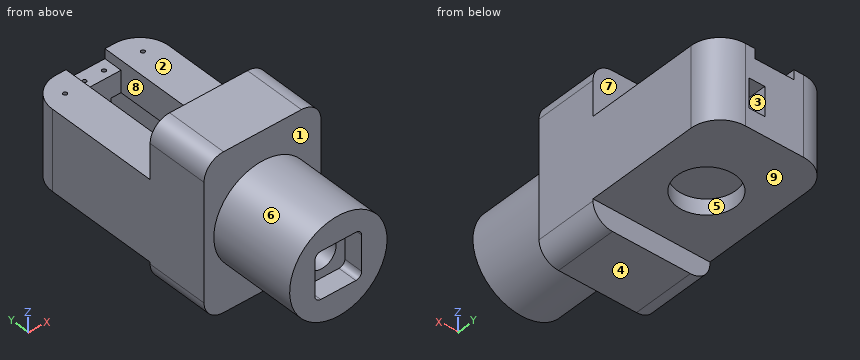
from build123d import *

# Parameters (mm, degrees)
SKETCH1_R                = 25
BOSS_EXTRUDE1_DEPTH      = 45
SKETCH2_W                = 60
SKETCH2_H                = 80
BOSS_EXTRUDE2_DEPTH      = 45
FILLET1_R                = 10
SKETCH3_W                = 60
SKETCH3_H                = 41
BOSS_EXTRUDE3_DEPTH      = 60
SKETCH4_W                = 20
SKETCH4_H                = 41
CUT_EXTRUDE1_DEPTH       = 32
SKETCH5_W                = 20
SKETCH5_H                = 9.5
CUT_EXTRUDE2_DEPTH       = 5
SKETCH7_R                = 15
CUT_EXTRUDE3_DEPTH       = 8
CUT_EXTRUDE4_REACH       = 163.567
SKETCH8_R                = 21
FILLET2_R                = 15
CUT_EXTRUDE5_REACH       = 169.812
SKETCH9_W                = 65
SKETCH9_H                = 65
CUT_EXTRUDE6_REACH       = 163.567
SKETCH10_W               = 65
SKETCH10_H               = 65
SKETCH11_R               = 1
CUT_EXTRUDE7_DEPTH       = 10
SKETCH12_R               = 1
CUT_EXTRUDE8_DEPTH       = 10
CUT_EXTRUDE9_START       = -27
SKETCH13_W               = 10
SKETCH13_H               = 9.5
CUT_EXTRUDE9_DEPTH       = 27
CUT_EXTRUDE10_DEPTH      = 5
CUT_EXTRUDE10_DEPTH_BACK = 3
SKETCH14_W               = 15
SKETCH14_H               = 62.680052408
SKETCH15_R               = 7.5
CUT_EXTRUDE11_DEPTH      = 90
SKETCH16_W               = 24
SKETCH16_H               = 24
CUT_EXTRUDE12_DEPTH      = 10
FILLET3_R                = 3


with BuildPart() as part:
    # Sketch1 → Boss-Extrude1 (new body)
    with BuildSketch(Plane(origin=(0, 0, 0), x_dir=(1, 0, 0), z_dir=(0, 1, 0))):
        with Locations(Location((0, 0, 0), (0, 0, 90))):
            Circle(SKETCH1_R)
    extrude(amount=BOSS_EXTRUDE1_DEPTH)

    # Sketch2 → Boss-Extrude2 (add)
    with BuildSketch(Plane(origin=(0, 45, 0), x_dir=(1, 0, 0), z_dir=(0, 1, 0))):
        Rectangle(SKETCH2_W, SKETCH2_H)
    extrude(amount=BOSS_EXTRUDE2_DEPTH)

    # Fillet1
    fillet1_edges = [part.edges().sort_by_distance(p)[0] for p in [
        (-30, 67.5, -40),
        (-30, 67.5, 40),
        (30, 67.5, 40),
        (30, 67.5, -40),
    ]]
    fillet(fillet1_edges, radius=FILLET1_R)

    # Sketch3 → Boss-Extrude3 (add)
    with BuildSketch(Plane(origin=(0, 90, 0), x_dir=(1, 0, 0), z_dir=(0, 1, 0))):
        with Locations((0, 8.5)):
            Rectangle(SKETCH3_W, SKETCH3_H)
    extrude(amount=BOSS_EXTRUDE3_DEPTH)

    # Sketch4 → Cut-Extrude1 (cut)
    with BuildSketch(Plane.XY.offset(12)):
        with Locations((0, 120)):
            Rectangle(SKETCH4_W, SKETCH4_H)
    extrude(amount=-CUT_EXTRUDE1_DEPTH, mode=Mode.SUBTRACT)

    # Sketch5 → Cut-Extrude2 (cut)
    with BuildSketch(Plane.XY.offset(12)):
        with Locations((0, 94.75)):
            Rectangle(SKETCH5_W, SKETCH5_H)
        with Locations((0, 145.25)):
            Rectangle(SKETCH5_W, SKETCH5_H)
    extrude(amount=-CUT_EXTRUDE2_DEPTH, mode=Mode.SUBTRACT)

    # Sketch7 → Cut-Extrude3 (cut)
    with BuildSketch(Plane(origin=(0, 0, -29), x_dir=(-1, 0, 0), z_dir=(0, 0, -1))):
        with Locations((0.1, 109.5)):
            Circle(SKETCH7_R)
    extrude(amount=-CUT_EXTRUDE3_DEPTH, mode=Mode.SUBTRACT)

    # Sketch8 → Cut-Extrude4 (cut, up to next)
    with BuildSketch(Plane.XY.offset(12), mode=Mode.PRIVATE) as cut_extrude4_sk1:
        with Locations((-0.1, 109.5)):
            Circle(SKETCH8_R)
    cut_extrude4_tool1 = extrude(cut_extrude4_sk1.sketch, amount=CUT_EXTRUDE4_REACH, mode=Mode.PRIVATE) & part.part
    add(cut_extrude4_tool1.solids().sort_by_distance((-0.1, 109.5, 12))[0], mode=Mode.SUBTRACT)

    # Fillet2
    fillet2_edges = [part.edges().sort_by_distance(p)[0] for p in [
        (-30, 150, -8.5),
        (30, 150, -8.5),
    ]]
    fillet(fillet2_edges, radius=FILLET2_R)

    # Sketch9 → Cut-Extrude5 (cut, up to next)
    with BuildSketch(Plane(origin=(0, 0, -29), x_dir=(-1, 0, 0), z_dir=(0, 0, -1)), mode=Mode.PRIVATE) as cut_extrude5_sk1:
        with Locations((0.1, 109.5)):
            Rectangle(SKETCH9_W, SKETCH9_H)
    cut_extrude5_tool1 = extrude(cut_extrude5_sk1.sketch, amount=CUT_EXTRUDE5_REACH, mode=Mode.PRIVATE) & part.part
    add(cut_extrude5_tool1.solids().sort_by_distance((-0.1, 109.5, -29))[0], mode=Mode.SUBTRACT)

    # Sketch10 → Cut-Extrude6 (cut, up to next)
    with BuildSketch(Plane.XY.offset(12), mode=Mode.PRIVATE) as cut_extrude6_sk1:
        with Locations((-0.1, 109.5)):
            Rectangle(SKETCH10_W, SKETCH10_H)
    cut_extrude6_tool1 = extrude(cut_extrude6_sk1.sketch, amount=CUT_EXTRUDE6_REACH, mode=Mode.PRIVATE) & part.part
    add(cut_extrude6_tool1.solids().sort_by_distance((-0.1, 109.5, 12))[0], mode=Mode.SUBTRACT)

    # Sketch11 → Cut-Extrude7 (cut)
    with BuildSketch(Plane.XY.offset(12)):
        with Locations((-20, 86)):
            Circle(SKETCH11_R)
        with Locations((20, 86)):
            Circle(SKETCH11_R)
        with Locations((20, 139)):
            Circle(SKETCH11_R)
        with Locations((-20, 139)):
            Circle(SKETCH11_R)
    extrude(amount=-CUT_EXTRUDE7_DEPTH, mode=Mode.SUBTRACT)

    # Sketch12 → Cut-Extrude8 (cut)
    with BuildSketch(Plane.XY.offset(7)):
        with Locations((4.9, 144.689613301)):
            Circle(SKETCH12_R)
        with Locations((-5.1, 144.689613301)):
            Circle(SKETCH12_R)
    extrude(amount=-CUT_EXTRUDE8_DEPTH, mode=Mode.SUBTRACT)

    # Sketch13 → Cut-Extrude9 (cut)
    with BuildSketch(Plane.XY.offset(7).offset(CUT_EXTRUDE9_START)):
        with Locations((0, 94.75)):
            Rectangle(SKETCH13_W, SKETCH13_H)
    extrude(amount=CUT_EXTRUDE9_DEPTH, mode=Mode.SUBTRACT)

    # Sketch14 → Cut-Extrude10 (cut, two sides: drawn at the far end of the back side and taken through both)
    with BuildSketch(Plane.ZY.offset(-10).offset(-CUT_EXTRUDE10_DEPTH_BACK)):
        with Locations((-11.671219496, 121.340026204)):
            Rectangle(SKETCH14_W, SKETCH14_H)
    extrude(amount=CUT_EXTRUDE10_DEPTH + CUT_EXTRUDE10_DEPTH_BACK, mode=Mode.SUBTRACT)

    # Sketch15 → Cut-Extrude11 (cut)
    with BuildSketch(Plane.XZ):
        with Locations(Location((0, 0, 0), (0, 0, 270))):
            Circle(SKETCH15_R)
    extrude(amount=-CUT_EXTRUDE11_DEPTH, mode=Mode.SUBTRACT)

    # Sketch16 → Cut-Extrude12 (cut)
    with BuildSketch(Plane.XZ):
        Rectangle(SKETCH16_W, SKETCH16_H)
    extrude(amount=-CUT_EXTRUDE12_DEPTH, mode=Mode.SUBTRACT)

    # Fillet3
    fillet3_edges = [part.edges().sort_by_distance(p)[0] for p in [
        (-12, 5, -12),
        (-12, 5, 12),
        (12, 5, 12),
        (12, 5, -12),
    ]]
    fillet(fillet3_edges, radius=FILLET3_R)


solid = part.part
Design review of the part built by this model. Coordinates are the model's own, in mm. Face numbers are marked on the shaded views. A direction names the side the tool comes from. Give positions to 0.01 mm unless a question says otherwise; leave off trailing zeros. Loops run counter-clockwise (first coordinate to the right, second up) from the corner with the lowest first, then second, coordinate; pieces in that order, holes last. Notation, with made-up numbers: (29.25, 5) -> (66.25, 5) arc R33 ccw to (66.25, 43) -> close; hole circle Ø1 at (10, 82). An arc over 180 degrees is marked (long way). One line per question, with ' | ' between items. Start each with the question number.
(1) We need section A-A (y = 51.5). State the section outline as (x, z) points, and give its area (3 significant figures).
(2) We need section D-D (x = 0). State the section outline as (y, z) points, and give its area (3 significant figures).
(3) Draft analysis for pull direction Z (two halves, no side actions). For the marked faces 1, 2, 3 and 4, state which applies: +Z half, -Z half, draft (parallel to the pull), parting line (faces both ways), or undercut.
(4) For line 1 (X direction, y = 86, z = 7.75); line 2 (Y direction, x = 0, z = -11); line 3 (Y direction, x = -0.1, z = -24.75), list the stretches that pass through material, from the lowest coordinate up.
(5) We need section C-C (y = 109.5). State the section outline as (x, z) points, and give its area (4 significant figures).
(6) Insertion check: P1, Ø1.8, axis at x = -20, y = 86, coming from the +Z side; P2, Ø1.5, axis at x = -5.5, y = 133.5, coming from the +Z side; P3, Ø2.5, axis at x = 4.9, y = 144.69, coming from the -Z side. Each pin has a flat end and moves straight along its axis. Give the tip position at first contact, or say it passes through.
(7) For the marked faces 5, 6, 7, 8 and 9, list the 3-axis set-ups (+Z, -Z, +X, -X, +Y, -Y) from which the entire face can be reached by the end or side of a thin tool; tool diameter is ignored.
(8) We need section B-B (z = 0). State the section outline as (x, y) points, and give its area (3 significant figures).
The answers:
1) outline: (-30, -30) arc R10 ccw to (-20, -40) -> (20, -40) arc R10 ccw to (30, -30) -> (30, 30) arc R10 ccw to (20, 40) -> (-20, 40) arc R10 ccw to (-30, 30) -> close; hole circle Ø15 at (0, 0) | area: 4,540 mm^2
2) outline: (0, -25) -> (45, -25) -> (45, -40) -> (77, -40) -> (77, -29) -> (94.5, -29) -> (94.5, -21) -> (124.5, -21) -> (124.5, -29) -> (150, -29) -> (150, 7) -> (140.5, 7) -> (140.5, -20) -> (90, -20) -> (90, -7.5) -> (10, -7.5) -> (10, -12) -> (0, -12) -> close; (0, 12) -> (10, 12) -> (10, 7.5) -> (90, 7.5) -> (90, 12) -> (77, 12) -> (77, 40) -> (45, 40) -> (45, 25) -> (0, 25) -> close | area: 4,460 mm^2
3) face 1: draft | face 2: +Z half | face 3: undercut | face 4: -Z half
4) line 1: x = -30 to -21, -19 to 19, 21 to 30 | line 2: y = 10 to 90, 140.5 to 150 | line 3: y = 0 to 94.5, 124.5 to 150
5) outline: (-30, -29) -> (-15.1, -29) -> (-15.1, -21) -> (14.9, -21) -> (14.9, -29) -> (30, -29) -> (30, 12) -> (10, 12) -> (10, -4.17) -> (13, -4.17) -> (13, -19.17) -> (10, -19.17) -> (10, -20) -> (-10, -20) -> (-10, 12) -> (-30, 12) -> close | area: 1,535 mm^2
6) P1: stops at z = 2 | P2: stops at z = -20 | P3: stops at z = -29
7) face 5: -Z | face 6: -Y | face 7: +Z, +X, -X, +Y | face 8: +Z | face 9: -Z, +X, -X, +Y
8) outline: (-30, 45) -> (-25, 45) -> (-25, 0) -> (-12, 0) -> (-12, 10) -> (-7.5, 10) -> (-7.5, 90) -> (-5, 90) -> (-5, 99.5) -> (-10, 99.5) -> (-10, 140.5) -> (10, 140.5) -> (10, 99.5) -> (5, 99.5) -> (5, 90) -> (7.5, 90) -> (7.5, 10) -> (12, 10) -> (12, 0) -> (25, 0) -> (25, 45) -> (30, 45) -> (30, 135) arc R15 ccw to (15, 150) -> (-15, 150) arc R15 ccw to (-30, 135) -> close; hole circle Ø2 at (-5.1, 144.69); hole circle Ø2 at (4.9, 144.69) | area: 6,090 mm^2
